from build123d import *

# Parameters (mm, degrees)
SKETCH1_R           = 1.9
SKETCH1_R_2         = 1.75
BOSS_EXTRUDE1_DEPTH = 5


with BuildPart() as part:
    # Sketch1 → Boss-Extrude1 (new body)
    with BuildSketch(Plane.XY):
        with BuildLine():
            Line((22.7, -12.5), (33.7, -12.5))
            ThreePointArc((33.7, -12.5), (34.407106781, -12.207106781), (34.7, -11.5))
            Line((34.7, -11.5), (34.7, 12.5))
            add(Edge.make_bspline(
                [(34.3, 17.348309182), (34.529755129, 14.926573724), (34.7, 12.5)],
                knots=[0, 0, 0, 1, 1, 1], degree=2))
            Line((34.3, 17.348309182), (34.3, 270.651690818))
            add(Edge.make_bspline(
                [(34.3, 270.651690818), (34.529755129, 273.073426276), (34.7, 275.5)],
                knots=[0, 0, 0, 1, 1, 1], degree=2))
            Line((34.7, 275.5), (34.7, 299.5))
            ThreePointArc((34.7, 299.5), (34.407106781, 300.207106781), (33.7, 300.5))
            Line((33.7, 300.5), (22.7, 300.5))
            Line((22.7, 300.5), (3, 300.5))
            ThreePointArc((3, 300.5), (1.585786438, 299.914213562), (1, 298.5))
            Line((1, 298.5), (1, 277.5))
            ThreePointArc((1, 277.5), (1.585786438, 276.085786438), (3, 275.5))
            Line((3, 275.5), (12.676771392, 275.5))
            add(Edge.make_bspline(
                [(23.1, 265.447646174), (20.336020381, 273.078870877), (12.676771392, 275.5)],
                knots=[0, 0, 0, 1, 1, 1], degree=2))
            Line((23.1, 265.447646174), (23.1, 22.552353826))
            add(Edge.make_bspline(
                [(23.1, 22.552353826), (20.336020381, 14.921129123), (12.676771392, 12.5)],
                knots=[0, 0, 0, 1, 1, 1], degree=2))
            Line((12.676771392, 12.5), (3, 12.5))
            ThreePointArc((3, 12.5), (1.585786438, 11.914213562), (1, 10.5))
            Line((1, 10.5), (1, -10.5))
            ThreePointArc((1, -10.5), (1.585786438, -11.914213562), (3, -12.5))
            Line((3, -12.5), (22.7, -12.5))
        make_face()
        with Locations((9.85, -10)):
            Circle(SKETCH1_R, mode=Mode.SUBTRACT)
        with Locations((9.85, 10)):
            Circle(SKETCH1_R_2, mode=Mode.SUBTRACT)
        with Locations((24.85, 10)):
            Circle(SKETCH1_R, mode=Mode.SUBTRACT)
        with Locations((24.85, -10)):
            Circle(SKETCH1_R, mode=Mode.SUBTRACT)
        with Locations((28.7, 131.5)):
            Circle(SKETCH1_R_2, mode=Mode.SUBTRACT)
        with Locations((28.7, 156.5)):
            Circle(SKETCH1_R_2, mode=Mode.SUBTRACT)
        with Locations((28.7, 256.5)):
            Circle(SKETCH1_R_2, mode=Mode.SUBTRACT)
        with Locations((28.7, 31.5)):
            Circle(SKETCH1_R_2, mode=Mode.SUBTRACT)
        with Locations(Location((24.85, 298, 0), (0, 0, 180))):
            Circle(SKETCH1_R, mode=Mode.SUBTRACT)
        with Locations(Location((24.85, 278, 0), (0, 0, 180))):
            Circle(SKETCH1_R, mode=Mode.SUBTRACT)
        with Locations(Location((9.85, 278, 0), (0, 0, 180))):
            Circle(SKETCH1_R_2, mode=Mode.SUBTRACT)
        with Locations(Location((9.85, 298, 0), (0, 0, 180))):
            Circle(SKETCH1_R, mode=Mode.SUBTRACT)
    extrude(amount=BOSS_EXTRUDE1_DEPTH)


solid = part.part
Design review of the part built by this model. Coordinates are the model's own, in mm. A direction names the side the tool comes from. Round coordinates to 2 decimals unless told otherwise and drop trailing zeros. Write each loop counter-clockwise with the first axis right and the second up, starting at its lowest first coordinate (ties: lowest second). Pieces come first, ordered by that corner, then holes.
Item 1: Consider section B-B on z = 1.9. Count the separate pieces of the cut face and the enclosed holes in it, and give its area (3 significant figures).
Item 2: Draft analysis for pull direction Y (two halves, no side actions). For faces 4 (the flat face through (1, 288, 2)), 5 (the flat face through (23.1, 146, 2)), 6 (the flat face through (19, 300.5, 2)), 7 (the flat face through (8, 12.5, 2)), state which applies: released by +Y, released by -Y, zero draft, split by the parting line, or undercut.
Item 3: Consider section A-A on y = 39.5. Give the boundary of the cut face in (x, z).
Item 4: For faces 1 (the flat face through (34.3, 142, 2)), 2 (the flat face through (8, 275.5, 2)), 3 (the flat face through (34.7, 287, 2)), list the 3-axis set-ups (+Z, -Z, +X, -X, +Y, -Y) from which the entire face can be reached by the end or side of a thin tool; tool diameter is ignored.
Item 5: For pin 1 Ø4.5 at (x, y) = (9.85, -10) entering from -Z; pin 2 Ø1.5 at (y, z) = (112.5, 2) entering from +X, all flat-tipped, find the tip position at first contact; note any pin that passes through.
Item 6: Wall thickness on L1, parallel to Y at x = 9.85, z = 2.4; L2, parallel to Y at x = 28.7, z = 3.5; L3, parallel to X at y = 278, z = 1.85: over which ranges is each line inside the solid? List them lowest first.
Check values:
1. separate pieces: 1
1. enclosed holes: 12
1. area: 4,570 mm2
2. face 4: zero draft
2. face 5: undercut
2. face 6: released by +Y
2. face 7: undercut
3. outline: (23.1, 0) - (34.3, 0) - (34.3, 5) - (23.1, 5) - close
4. face 1: +Z, -Z, +X
4. face 2: +Z, -Z, -X
4. face 3: +Z, -Z, +X, +Y, -Y
5. pin 1: stops at z = 0
5. pin 2: stops at x = 34.3
6. L1: y = -12.5 to -11.9, -8.1 to 8.25, 11.75 to 12.5, 275.5 to 276.25, 279.75 to 296.1, 299.9 to 300.5
6. L2: y = -12.5 to 29.75, 33.25 to 129.75, 133.25 to 154.75, 158.25 to 254.75, 258.25 to 300.5
6. L3: x = 1 to 8.1, 11.6 to 22.95, 26.75 to 34.7
